Input: part model. Units: mm. Frame: model coordinates. A direction names the side the tool comes from. Coordinates: 2 decimals unless noted, no trailing zeros. Write each loop counter-clockwise with the first axis right and the second up, starting at its lowest first coordinate (ties: lowest second). Pieces come first, ordered by that corner, then holes. Notation, with made-up numbers: M 86.25,-6.5 L 136.25,-6.5 A36 cw 136.25,32.5 Z; hole C 51.25,79.5 d8. An arc over 180 degrees is marked long. Use one line per item in the form item = value.
from build123d import *

# Parameters (mm, degrees)
SKETCH1_R           = 1
BOSS_EXTRUDE1_DEPTH = 3


with BuildPart() as part:
    # Sketch1 → Boss-Extrude1 (new body)
    with BuildSketch(Plane(origin=(0, 0, 0), x_dir=(1, 0, 0), z_dir=(0, 1, 0))):
        Polygon((2.309401077, 4), (-2.309401077, 4), (-4.618802154, 0), (-2.309401077, -4), (2.309401077, -4), (4.618802154, 0), align=None)
        Circle(SKETCH1_R, mode=Mode.SUBTRACT)
    extrude(amount=BOSS_EXTRUDE1_DEPTH)

    # Sketch2 → Revolve1 (revolve)
    with BuildSketch(Plane.XY):
        Polygon((2.5, 3), (1, 3), (1, 10.5), (3, 10.5), (3, 5), (2.5, 5), align=None)
        Polygon((1, 0), (2.000415076, 0), (0.6, -2), (0.225, -2), align=None)
    revolve(axis=Axis((0, -2, 0), (0, 1, 0)))


solid = part.part
(1) Section query B-B on x = -2.75. Return the cut outline in (y, z).
Computed:
outline = M 0,-3.24 L 3,-3.24 L 3,3.24 L 0,3.24 Z; M 5,-1.2 L 10.5,-1.2 L 10.5,1.2 L 5,1.2 Z
(2) Set-up query: faces 1 (the flat face through (-2, 5, -2)), 2 (the flat face through (1, 0, -2)), 3 (the flat face through (-3.48, 1.48, 1.97)). Return all of +Z, -Z, +X, -X, +Y, -Y with unobstructed straight access to the full face (end or side cutting, diameter ignored); none if empty.
Computed:
face_1 = none
face_2 = -Y
face_3 = +Z, -X, +Y, -Y
(3) Pull-direction query (X, two-part tool) for faces 4 (the cylindrical face through (0, 5, 1)), 5 (the flat face through (0, 1, -4)), 6 (the cylindrical face through (-3, 8, 0)); classes: pulls with the +X half, pulls with the -X half, needs draft (parallel to the pull), parting line crosses it, or undercut.
Computed:
face_4 = undercut
face_5 = needs draft
face_6 = parting line crosses it
(4) Line query: probe 1 along Z at (x, y) = (0, 7); probe 2 along Z at (x, y) = (0, 4.25). Output: solid intervals per line, ascending.
Computed:
probe_1 = -3 to -1, 1 to 3
probe_2 = -2.5 to -1, 1 to 2.5
(5) Section query C-C on z = 2.25. Return the cut outline in (x, y), plus the area to 3 significant figures.
Computed:
outline = M -3.32,0 L 3.32,0 L 3.32,3 L 1.09,3 L 1.09,5 L 1.98,5 L 1.98,10.5 L -1.98,10.5 L -1.98,5 L -1.09,5 L -1.09,3 L -3.32,3 Z
area = 46.1 mm^2
(6) First-contact query: pin 1 Ø1 at (x, y) = (-3, 5) entering from -Z; pin 2 Ø2 at (y, z) = (2, 1.5) entering from +X; pin 3 Ø1 at (y, z) = (4, 0.5) entering from +X. Flat tips, straight axial feed; report the tip coordinate or a pass-through.
Computed:
pin_1 = -1.66
pin_2 = 4.33
pin_3 = 2.5
(7) Section query D-D on x = 0. Return the cut outline in (y, z) (3 decimals), plus the area to 3 significant figures.
Computed:
outline = M -2,-0.6 L 0,-2 L 0,-4 L 3,-4 L 3,-2.5 L 5,-2.5 L 5,-3 L 10.5,-3 L 10.5,-1 L 0,-1 L -2,-0.225 Z; M -2,0.225 L 0,1 L 10.5,1 L 10.5,3 L 5,3 L 5,2.5 L 3,2.5 L 3,4 L 0,4 L 0,2 L -2,0.6 Z
area = 48.8 mm^2
(8) Section query A-A on y = 0.5. Return the cut outline in (x, z).
Computed:
outline = M -4.62,0 L -2.31,-4 L 2.31,-4 L 4.62,0 L 2.31,4 L -2.31,4 Z; hole C 0,0 d2
